Design review of the part shown in the three views and the two pictorial views. Dimensions are in mm from the part's minimum x, y and z. A direction names the side the tool comes from. Give positions to 0.01 mm unless a question says otherwise; leave off trailing zeros. Write each loop counter-clockwise with the first axis right and the second up, starting at its lowest first coordinate (ties: lowest second). Pieces come first, ordered by that corner, then holes. Notation, with made-up numbers: (4, -6.75) -> (48, -6.75) arc R32 ccw to (48, 23.25) -> close; hole circle Ø9 at (74.5, 70.5). An arc over 180 degrees is marked (long way). Use CSV: the item, a comma, the result in double quotes.
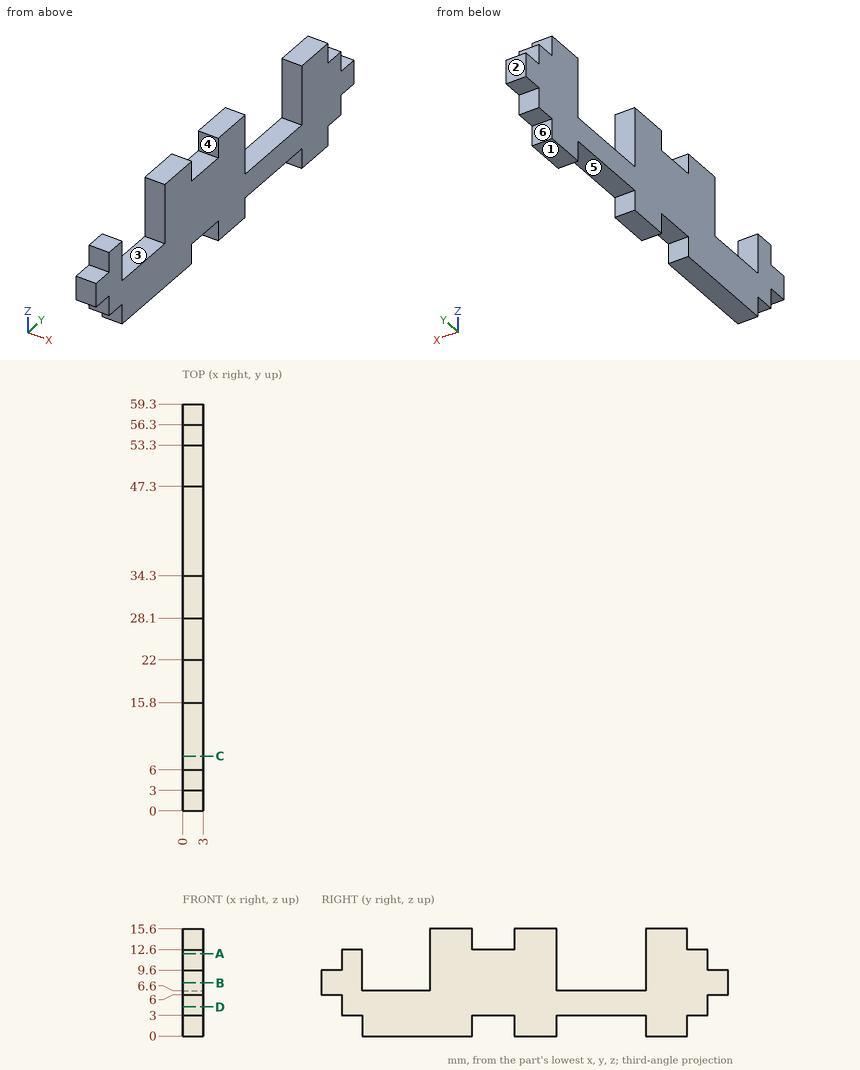
Q1. Insertion check: pin 1 (1.5 mm diameter, centred on x = 1, z = 10.5, fed in from +Y); pin 2 (1.5 mm diameter, centred on x = 1, z = 2, fed in from -Y); pin 3 (0.9 mm diameter, centred on x = 2, y = 23.5, fed in from +Z). Each pin has a flat end and moves straight along its axis. Give the tip position at first contact, or say it passes through.
Derived:
pin 1,"stops at y = 56.3"
pin 2,"stops at y = 6"
pin 3,"stops at z = 12.6"
Q2. Machinability: for the marked faces 4, 5 and 6, which of the approach directions +Z, -Z, +X, -X, +Y, -Y give a long, thin tool a straight path to every point of the face, cutting with its end or side? Answer none if there is none.
Derived:
face 4,"+Z, +X, -X"
face 5,"-Z, +X, -X"
face 6,"-Z, +X, -X, +Y"
Q3. Consider section D-D (z = 4.25). Write out the cut boundary in (x, y).
Derived:
outline,"(0, 3) -> (3, 3) -> (3, 56.3) -> (0, 56.3) -> close"
Q4. The part is to be moulded in two halves that separate along Y. For the marked faces 1, 2 and 3, say which applies: pulls with the +Y half, pulls with the -Y half, needs draft (parallel to the pull), parting line crosses it, or undercut.
Derived:
face 1,"needs draft"
face 2,"pulls with the +Y half"
face 3,"undercut"
Q5. Consider section A-A (z = 12). Write out the cut boundary in (x, y).
Derived:
outline,"(0, 3) -> (3, 3) -> (3, 6) -> (0, 6) -> close; (0, 15.8) -> (3, 15.8) -> (3, 34.3) -> (0, 34.3) -> close; (0, 47.3) -> (3, 47.3) -> (3, 56.3) -> (0, 56.3) -> close"
Q6. Consider section C-C (y = 8). Write out the cut boundary in (x, z), then the cut area to 3 significant figures.
Derived:
outline,"(0, 0) -> (3, 0) -> (3, 6.6) -> (0, 6.6) -> close"
area,"19.8 mm2"
Q7. Consider section B-B (z = 7.75). Write out the cut boundary in (x, y).
Derived:
outline,"(0, 0) -> (3, 0) -> (3, 6) -> (0, 6) -> close; (0, 15.8) -> (3, 15.8) -> (3, 34.3) -> (0, 34.3) -> close; (0, 47.3) -> (3, 47.3) -> (3, 59.3) -> (0, 59.3) -> close"
Q8. To check wall thickness, follow probe 1 along Y at (x, z) = (1.1, 13.25); probe 2 along Y at (x, z) = (2.65, 1.25); probe 3 along Z at (x, y) = (0.9, 15.5). State the ranges of each line that lie inside material, in increasing order.
Derived:
probe 1,"y = 15.8 to 22, 28.1 to 34.3, 47.3 to 53.3"
probe 2,"y = 6 to 22, 28.1 to 34.3, 47.3 to 53.3"
probe 3,"z = 0 to 6.6"
